Geometry: final body of the model. Coordinates: model frame, mm. Coordinates: 2 decimals unless noted, no trailing zeros. Loops run counter-clockwise (first coordinate to the right, second up) from the corner with the lowest first, then second, coordinate; pieces in that order, holes last. Notation, with made-up numbers: (43.5, -33) - (98.5, -33) arc R5 ccw to (98.5, -25) - close; hole circle Ø1 at (83.25, 22.5). An arc over 180 degrees is marked (long way). Put each result on its own line as item: value. Start each with the question number.
1) Section C-C on z = 33.5. Output: boundary loops of the cut face in (x, y) (3 decimals).
2) Contact query for flat-ended pins moving along their axis: pin 1 Ø1 at (x, y) = (12.5, 2) entering from +Z; pin 2 Ø1 at (y, z) = (2.5, -18.5) entering from +X. Output: stop coordinate, or through.
3) Section A-A on x = 47.5. Output: boundary loops of the cut face in (y, z) (3 decimals), and give its area (3 significant figures).
4) Material intervals for line 1 along X through (y, z) = (0.75, 0); line 2 along X through (y, z) = (2.4, -18.5); line 3 along X through (y, z) = (2.4, -5.5), sorted ascending. Write a range as from..to.
5) Section B-B on y = 2.5. Output: boundary loops of the cut face in (x, z) (3 decimals), and give its area (3 significant figures).
6) Section D-D on z = -27.5. Output: boundary loops of the cut face in (x, y) (3 decimals), and give its area (3 significant figures).
```python
from build123d import *

# Parameters (mm, degrees)
SKETCH1_W           = 152.4
SKETCH1_H           = 76.2
BOSS_EXTRUDE1_DEPTH = 3.175
CUT_EXTRUDE1_DEPTH  = 3.175
FILLET2_R           = 2.54
FILLET3_R           = 2.54
SKETCH5_R           = 7.62
CUT_EXTRUDE2_DEPTH  = 3.175
SKETCH7_R           = 1.0033
CUT_EXTRUDE4_DEPTH  = 86.253332046
SKETCH6_R           = 1.0033
CUT_EXTRUDE5_DEPTH  = 86.253332046


with BuildPart() as part:
    # Sketch1 → Boss-Extrude1 (new body)
    with BuildSketch(Plane(origin=(0, 0, 0), x_dir=(1, 0, 0), z_dir=(0, 1, 0))):
        Rectangle(SKETCH1_W, SKETCH1_H)
    extrude(amount=BOSS_EXTRUDE1_DEPTH)

    # Sketch4 → Cut-Extrude1 (cut)
    with BuildSketch(Plane(origin=(0, 3.175, 0), x_dir=(1, 0, 0), z_dir=(0, 1, 0))):
        with BuildLine():
            Line((0, 38.1), (76.2, 38.1))
            Line((76.2, 38.1), (76.2, 12.7))
            ThreePointArc((76.2, 12.7), (40.160926284, 31.582778852), (0, 38.1))
        make_face()
        with BuildLine():
            Line((76.2, -38.1), (76.2, -12.7))
            ThreePointArc((76.2, -12.7), (40.160926284, -31.582778852), (0, -38.1))
            Line((0, -38.1), (76.2, -38.1))
        make_face()
    extrude(amount=-CUT_EXTRUDE1_DEPTH, mode=Mode.SUBTRACT)

    # Fillet2
    fillet2_edges = [part.edges().sort_by_distance(p)[0] for p in [
        (76.2, 1.5875, -12.7),
        (76.2, 1.5875, 12.7),
    ]]
    fillet(fillet2_edges, radius=FILLET2_R)

    # Fillet3
    fillet3_edges = [part.edges().sort_by_distance(p)[0] for p in [
        (-76.2, 1.5875, -38.1),
        (-76.2, 1.5875, 38.1),
    ]]
    fillet(fillet3_edges, radius=FILLET3_R)

    # Sketch5 → Cut-Extrude2 (cut)
    with BuildSketch(Plane(origin=(0, 3.175, 0), x_dir=(1, 0, 0), z_dir=(0, 1, 0))):
        with Locations(Location((50.8, 0, 0), (0, 0, 270))):
            Circle(SKETCH5_R)
    extrude(amount=-CUT_EXTRUDE2_DEPTH, mode=Mode.SUBTRACT)

    # Sketch7 → Cut-Extrude4 (cut, through all)
    with BuildSketch(Plane(origin=(0, 3.175, 0), x_dir=(1, 0, 0), z_dir=(0, 1, 0))):
        with Locations(Location((70.485, 0, 0), (0, 0, 270))):
            Circle(SKETCH7_R)
        with Locations(Location((31.115, 0, 0), (0, 0, 270))):
            Circle(SKETCH7_R)
    extrude(amount=-CUT_EXTRUDE4_DEPTH, mode=Mode.SUBTRACT)

    # Sketch6 → Cut-Extrude5 (cut, through all)
    with BuildSketch(Plane(origin=(0, 3.175, 0), x_dir=(1, 0, 0), z_dir=(0, 1, 0))):
        with Locations(Location((-63.5, 18.542, 0), (0, 0, 270))):
            Circle(SKETCH6_R)
        with Locations(Location((-24.13, 18.542, 0), (0, 0, 270))):
            Circle(SKETCH6_R)
        with Locations(Location((-24.13, -18.542, 0), (0, 0, 270))):
            Circle(SKETCH6_R)
        with Locations(Location((-63.5, -18.542, 0), (0, 0, 270))):
            Circle(SKETCH6_R)
    extrude(amount=-CUT_EXTRUDE5_DEPTH, mode=Mode.SUBTRACT)


solid = part.part
```
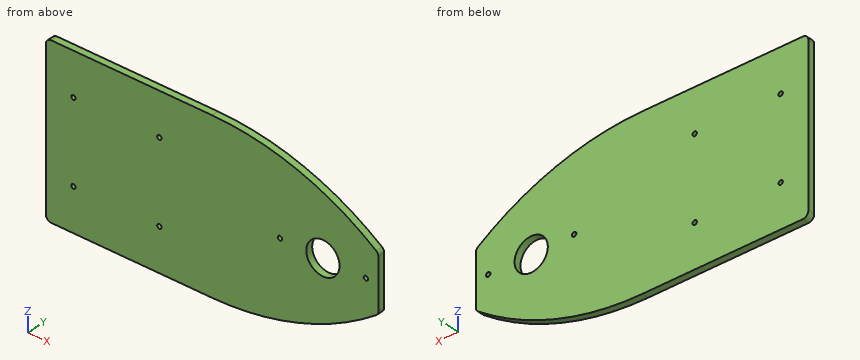
Answer block:
1. outline: (-76.2, 0) - (33.871, 0) - (33.871, 3.175) - (-76.2, 3.175) - close
2. pin 1: stops at z = 37.53
2. pin 2: stops at x = 68.57
3. outline: (0, -28.883) - (3.175, -28.883) - (3.175, -6.868) - (0, -6.868) - close; (0, 6.868) - (3.175, 6.868) - (3.175, 28.883) - (0, 28.883) - close
3. area: 140 mm²
4. line 1: x = -76.2..30.11, 32.12..43.18, 58.42..69.48, 71.49..76.2
4. line 2: x = -76.2..-64.5, -62.5..-25.13, -23.13..67.78
4. line 3: x = -76.2..45.53, 56.07..76.2
5. outline: (-76.2, -35.56) arc R2.54 ccw to (-73.66, -38.1) - (0, -38.1) arc R127 ccw to (75.163, -13.469) arc R2.54 ccw to (76.2, -11.422) - (76.2, 11.422) arc R2.54 ccw to (75.163, 13.469) arc R127 ccw to (0, 38.1) - (-73.66, 38.1) arc R2.54 ccw to (-76.2, 35.56) - close; hole circle Ø2.007 at (-63.5, -18.542); hole circle Ø2.007 at (-63.5, 18.542); hole circle Ø2.007 at (-24.13, -18.542); hole circle Ø2.007 at (-24.13, 18.542); hole circle Ø2.007 at (31.115, 0); hole circle Ø15.24 at (50.8, 0); hole circle Ø2.007 at (70.485, 0)
5. area: 10,200 mm²
6. outline: (-76.2, 0) - (50.794, 0) - (50.794, 3.175) - (-76.2, 3.175) - close
6. area: 403 mm²
